Design review of the part built by this model. Coordinates are the model's own, in mm. Coordinates: 2 decimals unless noted, no trailing zeros. Loops run counter-clockwise (first coordinate to the right, second up) from the corner with the lowest first, then second, coordinate; pieces in that order, holes last. Notation, with made-up numbers: (-1, 29.25) - (28, 29.25) arc R20 cw to (28, 53.25) - close; hole circle Ø3 at (34, 29). An arc over 180 degrees is marked (long way). Return JSON: item names as keys, results as strings. Group by question number.
from build123d import *

# Parameters (mm, degrees)
SKETCH1_R           = 2.5
SKETCH1_R_2         = 3
BOSS_EXTRUDE1_DEPTH = 3
CHAMFER_1_SIZE      = 0.2


with BuildPart() as part:
    # Sketch1 → Boss-Extrude1 (new, symmetric)
    with BuildSketch(Plane.XY):
        with BuildLine():
            Line((0, 5), (50, 5))
            ThreePointArc((50, 5), (55, 0), (50, -5))
            Line((50, -5), (0, -5))
            ThreePointArc((0, -5), (-5, 0), (0, 5))
        make_face()
        with Locations((50, 0)):
            Circle(SKETCH1_R, mode=Mode.SUBTRACT)
        Circle(SKETCH1_R_2, mode=Mode.SUBTRACT)
    extrude(amount=BOSS_EXTRUDE1_DEPTH, both=True)

    # 倒角1
    chamfer_1_edges = [part.edges().sort_by_distance(p)[0] for p in [
        (47.5, 0, -3),
        (47.5, 0, 3),
        (-3, 0, -3),
        (-3, 0, 3),
    ]]
    chamfer(chamfer_1_edges, length=CHAMFER_1_SIZE)


solid = part.part
Item 1: Add section A-A (y = 0). State the section outline as (x, z) points, then the cut area to 3 significant figures.
Item 2: Draft analysis for pull direction Y (two halves, no side actions). For faces 1 (the face through (52.31, -0.96, -0.04)), 2 (the face through (55, 0, 0)), 3 (the face through (-3, 0, 0)), 4 (the face through (25, 0, 3)), state which applies: pulls with the +Y half, pulls with the -Y half, needs draft (parallel to the pull), parting line crosses it, or undercut.
Item 3: For P1, Ø1.5, axis at y = -4, z = 0, coming from the -X side; P2, Ø2, axis at y = 1.5, z = -2, coming from the -X side, all flat-tipped, find the tip position at first contact; note any pin that passes through.
Item 4: Add section B-B (z = -0.7). State the section outline as (x, y) points, then the cut area to 3 significant figures.
Item 5: To check wall thickness, follow line 1 (Y direction, x = 50, z = -0.5); line 2 (X direction, y = -2.25, z = 2.2); line 3 (X direction, y = 1, z = 0.6). State the ranges of each line that lie inside material, in increasing order. Write a range as from..to.
Answers below:
{
 "1": {"outline": "(-5, -3) - (-3.2, -3) - (-3, -2.8) - (-3, 2.8) - (-3.2, 3) - (-5, 3) - close; (3, -2.8) - (3.2, -3) - (47.3, -3) - (47.5, -2.8) - (47.5, 2.8) - (47.3, 3) - (3.2, 3) - (3, 2.8) - close; (52.5, -2.8) - (52.7, -3) - (55, -3) - (55, 3) - (52.7, 3) - (52.5, 2.8) - close", "area": "294 mm^2"},
 "2": {"face 1": "undercut", "face 2": "parting line crosses it", "face 3": "undercut", "face 4": "needs draft"},
 "3": {"P1": "stops at x = -3.8", "P2": "stops at x = -4.97"},
 "4": {"outline": "(0, -5) - (50, -5) arc R5 ccw to (50, 5) - (0, 5) arc R5 ccw to start; hole circle Ø6 at (0, 0); hole circle Ø5 at (50, 0)", "area": "531 mm^2"},
 "5": {"line 1": "y = -5..-2.5, 2.5..5", "line 2": "x = -4.47..-1.98, 1.98..48.91, 51.09..54.47", "line 3": "x = -4.9..-2.83, 2.83..47.71, 52.29..54.9"}
}
